```python
from build123d import *

# Parameters (mm, degrees)
SKETCH1_W           = 34.5
SKETCH1_H           = 25.9
SKETCH1_R           = 1.55
BOSS_EXTRUDE1_DEPTH = 1.5
SKETCH3_W           = 34.5
SKETCH3_H           = 25.9
SKETCH3_R           = 2.25
BOSS_EXTRUDE3_DEPTH = 1.6
SKETCH5_W           = 34.5
SKETCH5_H           = 25.9
BOSS_EXTRUDE4_DEPTH = 1.8
SKETCH6_W           = 15.150257738
SKETCH6_H           = 1.5
BOSS_EXTRUDE5_DEPTH = 1.8
BOSS_EXTRUDE6_DEPTH = 1.5
CUT_EXTRUDE1_REACH  = 24.165
FILLET1_R           = 1.5
FILLET2_R           = 2.25


with BuildPart() as part:
    # Sketch1 → Boss-Extrude1 (new body)
    with BuildSketch(Plane(origin=(0, 0, 0), x_dir=(1, 0, 0), z_dir=(0, 1, 0))):
        Rectangle(SKETCH1_W, SKETCH1_H)
        with Locations(Location((-10, 10, 0), (0, 0, 270))):
            Circle(SKETCH1_R, mode=Mode.SUBTRACT)
        with Locations(Location((10, 10, 0), (0, 0, 270))):
            Circle(SKETCH1_R, mode=Mode.SUBTRACT)
        with Locations(Location((10, -10, 0), (0, 0, 270))):
            Circle(SKETCH1_R, mode=Mode.SUBTRACT)
        with Locations(Location((-10, -10, 0), (0, 0, 270))):
            Circle(SKETCH1_R, mode=Mode.SUBTRACT)
    extrude(amount=BOSS_EXTRUDE1_DEPTH)

    # Sketch3 → Boss-Extrude3 (add)
    with BuildSketch(Plane(origin=(0, 1.5, 0), x_dir=(1, 0, 0), z_dir=(0, 1, 0))):
        Rectangle(SKETCH3_W, SKETCH3_H)
        with Locations(Location((-10, 10, 0), (0, 0, 270))):
            Circle(SKETCH3_R, mode=Mode.SUBTRACT)
        with Locations(Location((10, 10, 0), (0, 0, 270))):
            Circle(SKETCH3_R, mode=Mode.SUBTRACT)
        with Locations(Location((10, -10, 0), (0, 0, 270))):
            Circle(SKETCH3_R, mode=Mode.SUBTRACT)
        with Locations(Location((-10, -10, 0), (0, 0, 270))):
            Circle(SKETCH3_R, mode=Mode.SUBTRACT)
    extrude(amount=BOSS_EXTRUDE3_DEPTH)

    # Sketch5 → Boss-Extrude4 (add)
    with BuildSketch(Plane(origin=(0, 3.1, 0), x_dir=(1, 0, 0), z_dir=(0, 1, 0))):
        Rectangle(SKETCH5_W, SKETCH5_H)
        with BuildLine():
            Line((-6, -10.95), (-6, -10))
            ThreePointArc((-6, -10), (-7.171572875, -7.171572875), (-10, -6))
            Line((-10, -6), (-15.25, -6))
            Line((-15.25, -6), (-15.25, 6))
            Line((-15.25, 6), (-10, 6))
            ThreePointArc((-10, 6), (-7.171572875, 7.171572875), (-6, 10))
            Line((-6, 10), (-6, 10.95))
            Line((-6, 10.95), (6, 10.95))
            Line((6, 10.95), (6, 10))
            ThreePointArc((6, 10), (7.171572875, 7.171572875), (10, 6))
            Line((10, 6), (15.25, 6))
            Line((15.25, 6), (15.25, -6))
            Line((15.25, -6), (10, -6))
            ThreePointArc((10, -6), (7.171572875, -7.171572875), (6, -10))
            Line((6, -10), (6, -10.95))
            Line((6, -10.95), (-6, -10.95))
        make_face(mode=Mode.SUBTRACT)
        Polygon((12.424871131, 10), (11.212435565, 7.9), (8.787564435, 7.9), (7.575128869, 10), (8.787564435, 12.1), (11.212435565, 12.1), align=None, mode=Mode.SUBTRACT)
        Polygon((-7.575128869, 10), (-8.787564435, 7.9), (-11.212435565, 7.9), (-12.424871131, 10), (-11.212435565, 12.1), (-8.787564435, 12.1), align=None, mode=Mode.SUBTRACT)
        Polygon((7.575128869, -10), (8.787564435, -7.9), (11.212435565, -7.9), (12.424871131, -10), (11.212435565, -12.1), (8.787564435, -12.1), align=None, mode=Mode.SUBTRACT)
        Polygon((-8.787564435, -12.1), (-11.212435565, -12.1), (-12.424871131, -10), (-11.212435565, -7.9), (-8.787564435, -7.9), (-7.575128869, -10), align=None, mode=Mode.SUBTRACT)
    extrude(amount=BOSS_EXTRUDE4_DEPTH)

    # Sketch6 → Boss-Extrude5 (add)
    with BuildSketch(Plane(origin=(0, 4.9, 0), x_dir=(1, 0, 0), z_dir=(0, 1, 0))):
        Polygon((-12.424871131, -11.45), (-15.75, -11.45), (-15.75, 11.45), (-12.424871131, 11.45), (-12.424871131, 12.95), (-17.25, 12.95), (-17.25, -12.95), (-12.424871131, -12.95), align=None)
        with Locations((0, 12.2)):
            Rectangle(SKETCH6_W, SKETCH6_H)
        Polygon((15.75, -11.45), (12.424871131, -11.45), (12.424871131, -12.95), (17.25, -12.95), (17.25, 12.95), (12.424871131, 12.95), (12.424871131, 11.45), (15.75, 11.45), align=None)
        with Locations((0, -12.2)):
            Rectangle(SKETCH6_W, SKETCH6_H)
    extrude(amount=BOSS_EXTRUDE5_DEPTH)

    # Sketch7 → Boss-Extrude6 (add)
    with BuildSketch(Plane(origin=(0, 6.7, 0), x_dir=(1, 0, 0), z_dir=(0, 1, 0))):
        Polygon((-13.75, 12.95), (-17.25, 12.95), (-17.25, 9.45), (-15.75, 9.45), (-15.75, 11.45), (-13.75, 11.45), align=None)
        Polygon((-13.75, 10.7), (-13.75, 11.45), (-15.75, 11.45), (-15.75, 9.45), (-15, 9.45), (-15, 10.7), align=None)
        Polygon((-15.75, -9.45), (-17.25, -9.45), (-17.25, -12.95), (-13.75, -12.95), (-13.75, -11.45), (-15.75, -11.45), align=None)
        Polygon((-15, -9.45), (-15.75, -9.45), (-15.75, -11.45), (-13.75, -11.45), (-13.75, -10.7), (-15, -10.7), align=None)
        Polygon((17.25, -12.95), (17.25, -9.45), (15, -9.45), (15, -10.7), (15, -12.95), align=None)
    extrude(amount=BOSS_EXTRUDE6_DEPTH)

    # Sketch8 → Cut-Extrude1 (cut, up to next)
    with BuildSketch(Plane(origin=(0, 3.1, 0), x_dir=(1, 0, 0), z_dir=(0, 1, 0)), mode=Mode.PRIVATE) as cut_extrude1_sk1:
        with BuildLine():
            Line((10, -6), (15.25, -6))
            Line((15.25, -6), (15.25, 6))
            Line((15.25, 6), (10, 6))
            ThreePointArc((10, 6), (7.171572875, 7.171572875), (6, 10))
            Line((6, 10), (6, 10.95))
            Line((6, 10.95), (-6, 10.95))
            Line((-6, 10.95), (-6, 10))
            ThreePointArc((-6, 10), (-7.171572875, 7.171572875), (-10, 6))
            Line((-10, 6), (-15.25, 6))
            Line((-15.25, 6), (-15.25, -6))
            Line((-15.25, -6), (-10, -6))
            ThreePointArc((-10, -6), (-7.171572875, -7.171572875), (-6, -10))
            Line((-6, -10), (-6, -10.95))
            Line((-6, -10.95), (6, -10.95))
            Line((6, -10.95), (6, -10))
            ThreePointArc((6, -10), (7.171572875, -7.171572875), (10, -6))
        make_face()
    cut_extrude1_tool1 = extrude(cut_extrude1_sk1.sketch, amount=-CUT_EXTRUDE1_REACH, mode=Mode.PRIVATE) & part.part
    add(cut_extrude1_tool1.solids().sort_by_distance((0, 3.1, 0))[0], mode=Mode.SUBTRACT)

    # Fillet1
    # the kernel refuses this fillet: 1.5 mm, written as the material it adds along each edge
    with BuildSketch(Plane(origin=(6, 4.9, 10.95), x_dir=(-1, 0, 0), z_dir=(0, -1, 0))) as fillet1_piece_1:
        with BuildLine():
            CenterArc((1.472430904, 1.5), FILLET1_R, 185.739170477, 84.260829523)
            Line((-0.020050252, 1.35), (-0.169298367, 1.335))
            ThreePointArc((-0.169298367, 1.335), (-0.15, 0.95), (-0.15, 0))
            Line((-0.15, 0), (0, -0.15))
            Line((0, -0.15), (1.472430904, -0.15))
            Line((1.472430904, -0.15), (1.472430904, 0))
        make_face()
    extrude(amount=4.9)
    with BuildSketch(Plane(origin=(15.25, 4.9, 6), x_dir=(-1, 0, 0), z_dir=(0, -1, 0)), Plane(origin=(15.25, 4.9, -6), x_dir=(0, 0, 1), z_dir=(0, -1, 0))) as fillet1_piece_2:
        with BuildLine():
            CenterArc((FILLET1_R, FILLET1_R), FILLET1_R, 180, 90)
            Line((0, FILLET1_R), (0, 0))
            Line((0, 0), (FILLET1_R, 0))
        make_face()
    extrude(amount=4.9)
    with BuildSketch(Plane(origin=(6, 4.9, -10.95), x_dir=(0.014850400419695863, 0, 0.9998897267235897), z_dir=(0, -1, 0))) as fillet1_piece_3:
        with BuildLine():
            CenterArc((1.477968402, 1.494544135), FILLET1_R, 180.850896545, 84.260829523)
            Line((-0.021866189, 1.472268534), (-0.171849648, 1.470040974))
            Line((-0.171849648, 1.470040974), (-0.149983459, -0.00222756))
            Line((-0.149983459, -0.00222756), (0.00222756, -0.149983459))
            ThreePointArc((0.00222756, -0.149983459), (0.9521228, -0.135875579), (1.337366934, -0.149454413))
            Line((1.337366934, -0.149454413), (1.350148885, 0))
        make_face()
    extrude(amount=4.9)
    with BuildSketch(Plane(origin=(-6, 0, -10.95), x_dir=(1, 0, 0), z_dir=(0, 1, 0))) as fillet1_piece_4:
        with BuildLine():
            CenterArc((1.472430904, -1.5), FILLET1_R, 90, 84.260829523)
            Line((-0.020050252, -1.35), (-0.169298367, -1.335))
            ThreePointArc((-0.169298367, -1.335), (-0.15, -0.95), (-0.15, 0))
            Line((-0.15, 0), (0, 0.15))
            Line((0, 0.15), (1.472430904, 0.15))
            Line((1.472430904, 0.15), (1.472430904, 0))
        make_face()
    extrude(amount=4.9)
    with BuildSketch(Plane(origin=(-15.25, 0, -6), x_dir=(1, 0, 0), z_dir=(0, 1, 0)), Plane(origin=(-15.25, 0, 6), x_dir=(0, 0, -1), z_dir=(0, 1, 0))) as fillet1_piece_5:
        with BuildLine():
            CenterArc((FILLET1_R, -FILLET1_R), FILLET1_R, 90, 90)
            Line((0, -FILLET1_R), (0, 0))
            Line((0, 0), (FILLET1_R, 0))
        make_face()
    extrude(amount=4.9)
    with BuildSketch(Plane(origin=(-6, 0, 10.95), x_dir=(-0.014850400419695205, 0, -0.9998897267235897), z_dir=(0, 1, 0))) as fillet1_piece_6:
        with BuildLine():
            CenterArc((1.477968402, -1.494544135), FILLET1_R, 94.888273932, 84.260829523)
            Line((-0.021866189, -1.472268534), (-0.171849648, -1.470040974))
            Line((-0.171849648, -1.470040974), (-0.149983459, 0.00222756))
            Line((-0.149983459, 0.00222756), (0.00222756, 0.149983459))
            ThreePointArc((0.00222756, 0.149983459), (0.9521228, 0.135875579), (1.337366934, 0.149454413))
            Line((1.337366934, 0.149454413), (1.350148885, 0))
        make_face()
    extrude(amount=4.9)
    with BuildSketch(Plane(origin=(17.25, 6.7, 9.45), x_dir=(0, 0, -1), z_dir=(-1, 0, 0)), Plane(origin=(15, 6.7, 11.45), x_dir=(-1, 0, 0), z_dir=(0, 0, 1)), Plane(origin=(-15.75, 6.7, 9.45), x_dir=(0, 0, -1), z_dir=(-1, 0, 0)), Plane(origin=(-15.75, 6.7, -9.45), x_dir=(0, 1, 0), z_dir=(-1, 0, 0))) as fillet1_piece_7:
        with BuildLine():
            CenterArc((FILLET1_R, -FILLET1_R), FILLET1_R, 90, 90)
            Line((0, -FILLET1_R), (0, 0))
            Line((0, 0), (FILLET1_R, 0))
        make_face()
    extrude(amount=1.5)
    with BuildSketch(Plane(origin=(-13.75, 6.7, -11.45), x_dir=(1, 0, 0), z_dir=(0, 0, -1))) as fillet1_piece_8:
        with BuildLine():
            CenterArc((1.5, -1.489771824), FILLET1_R, 96.694808908, 83.305191092)
            Line((0, -1.489771824), (0, 0))
            Line((0, 0), (1.325128869, 0))
        make_face()
    extrude(amount=1.5)
    with BuildSketch(Plane(origin=(-13.75, 6.7, 11.45), x_dir=(0, 1, 0), z_dir=(0, 0, 1))) as fillet1_piece_9:
        with BuildLine():
            CenterArc((1.489771824, -1.5), FILLET1_R, 90, 83.305191092)
            Line((0, -1.325128869), (0, 0))
            Line((0, 0), (1.489771824, 0))
        make_face()
    extrude(amount=1.5)

    # Fillet2
    fillet2_edges = [part.edges().sort_by_distance(p)[0] for p in [
        (17.25, 4.1, 12.95),
        (-17.25, 4.1, 12.95),
        (-17.25, 4.1, -12.95),
        (17.25, 3.35, -12.95),
    ]]
    fillet(fillet2_edges, radius=FILLET2_R)


solid = part.part
```
Read the model definition and answer for the solid it produces. Units are mm, in the model's axes. A direction names the side the tool comes from. Give positions to 0.01 mm unless a question says otherwise; leave off trailing zeros. Loops run counter-clockwise (first coordinate to the right, second up) from the corner with the lowest first, then second, coordinate; pieces in that order, holes last.
Item 1: The part is cut by section B-B (y = 2.5). Give the number of separate pieces and of enclosed holes in the cut face, and give its area (3 significant figures).
Item 2: Find the intervals of material crossed by line 1 along Z through (x, y) = (-10, 1.8); line 2 along Z through (x, y) = (10.5, 4.5); line 3 along Z through (x, y) = (13.5, 3.75), in increasing order.
Item 3: For faces 4 (the flat face through (10, 4, 7.9)), 5 (the cylindrical face through (7.29, 2.48, 7.06)), 6 (the flat face through (12.425, 6, 12)), determine the directions among +Z, -Z, +X, -X, +Y, -Y from which every point of the face is accessible in a straight line to the end or side of a thin tool.
Item 4: Each of these flat-tipped pins is pushed along its axis until it touches: pin 1 Ø4 at (x, z) = (10, -10) entering from +Y; pin 2 Ø3.5 at (x, z) = (10, 9) entering from +Y. Where does it stop, or does it pass through?
Item 5: The mould has two halves that part along X. Classify faces 1 (the flat face through (-16, 8.2, 11)), 2 (the flat face through (-15, 7, -10)), 3 (the flat face through (-15, 6.7, -11)): released by +X, released by -X, zero draft, split by the parting line, or undercut.
Item 6: The part is cut by section A-A (y = 6). Write down the section's boundary in (x, z).
Item 7: The part is cut by section D-D (x = -7). Write down the section's boundary in (y, z).
Item 8: The part is cut by section C-C (x = 2.5). Write down the section's boundary in (y, z).
Taken from the geometry:
1. separate pieces: 1
1. enclosed holes: 5
1. area: 331 mm2
2. line 1: z = -12.95 to -12.25, -7.75 to -6, 6 to 7.75, 12.25 to 12.95
2. line 2: z = -12.95 to -12.1, -7.9 to -6, 6 to 7.9, 12.1 to 12.95
2. line 3: z = -12.95 to -6, 6 to 12.95
3. face 4: +Y
3. face 5: +Y, -Y
3. face 6: +Z, -Z, +Y
4. pin 1: stops at y = 1.5
4. pin 2: stops at y = 4.9
5. face 1: zero draft
5. face 2: released by +X
5. face 3: undercut
6. outline: (-17.25, -10.7) arc R2.25 ccw to (-15, -12.95) - (-12.42, -12.95) - (-12.42, -11.45) - (-15.75, -11.45) - (-15.75, 11.45) - (-12.42, 11.45) - (-12.42, 12.95) - (-15, 12.95) arc R2.25 ccw to (-17.25, 10.7) - close; (-7.58, -12.95) - (7.58, -12.95) - (7.58, -11.45) - (-7.58, -11.45) - close; (-7.58, 11.45) - (7.58, 11.45) - (7.58, 12.95) - (-7.58, 12.95) - close; (12.42, -12.95) - (15, -12.95) arc R2.25 ccw to (17.25, -10.7) - (17.25, 10.7) arc R2.25 ccw to (15, 12.95) - (12.42, 12.95) - (12.42, 11.45) - (15.75, 11.45) - (15.75, -11.45) - (12.42, -11.45) - close
7. outline: (0, -12.95) - (6.7, -12.95) - (6.7, -11.45) - (4.9, -11.45) - (4.9, -7.35) - (0, -7.35) - close; (0, 7.35) - (4.9, 7.35) - (4.9, 11.45) - (6.7, 11.45) - (6.7, 12.95) - (0, 12.95) - close
8. outline: (0, -12.95) - (6.7, -12.95) - (6.7, -11.45) - (4.9, -11.45) - (4.9, -10.95) - (0, -10.95) - close; (0, 10.95) - (4.9, 10.95) - (4.9, 11.45) - (6.7, 11.45) - (6.7, 12.95) - (0, 12.95) - close
